from build123d import *

# Parameters (mm, degrees)
SKETCH_1_W          = 9.5
SKETCH_1_H          = 9.5
EXTRUDE_1_DEPTH     = 3
CUT_EXTRUDE_1_DEPTH = 1


with BuildPart() as part:
    # 草图1 → 凸台-拉伸1 (new body, symmetric)
    with BuildSketch(Plane.XY):
        with BuildLine():
            Line((-12, 0), (-12, 120))
            ThreePointArc((-12, 120), (0, 132), (12, 120))
            Line((12, 120), (12, 0))
            ThreePointArc((12, 0), (0, -12), (-12, 0))
        make_face()
        Rectangle(SKETCH_1_W, SKETCH_1_H, mode=Mode.SUBTRACT)
    extrude(amount=EXTRUDE_1_DEPTH, both=True)

    # 草图2 → 切除-拉伸1 (cut)
    with BuildSketch(Plane.XY.offset(3)):
        with BuildLine():
            Line((-6, 20), (-6, 120))
            ThreePointArc((-6, 120), (0, 126), (6, 120))
            Line((6, 120), (6, 20))
            ThreePointArc((6, 20), (0, 14), (-6, 20))
        make_face()
    cut_extrude_1 = extrude(amount=-CUT_EXTRUDE_1_DEPTH, mode=Mode.SUBTRACT)

    # 镜向1: 切除-拉伸1 across plane
    add(cut_extrude_1.mirror(Plane.XY), mode=Mode.SUBTRACT)


solid = part.part
The listing builds one solid part. Answer for the finished solid, in the listing's coordinates (mm). A direction names the side the tool comes from. Round coordinates to 2 decimals unless told otherwise and drop trailing zeros. Order: outer loops, then holes, each group sorted by start corner. A loop starts at its lowest first (then second) coordinate and runs counter-clockwise, first axis right, second up. Notation, with made-up numbers: (63, 88.5) - (73, 88.5) arc R12 ccw to (73, 98.5) - close; hole circle Ø1 at (73, -9.75). An arc over 180 degrees is marked (long way). Write item = value, one per line. Start each with the question number.
1) For a pull along X with two mould halves and no side action, classify faces 6 (the flat face through (-12, 59, 0)), 7 (the flat face through (0, 71, -2)), 8 (the flat face through (8, 61, -3)) as released by +X, released by -X, zero draft, split by the parting line, or undercut.
2) Given pin 1 (3.5 mm diameter, centred on x = -1, y = 55, fed in from +Z); pin 2 (5 mm diameter, centred on x = -5, y = 67, fed in from -Z); pin 3 (1 mm diameter, centred on x = -6, z = 2, fed in from -Y), each flat-ended and moving along its own axis, determine where each tip first touches the part or whether it passes through.
3) Section B-B, the plane x = 0 is taken. Write down the section's boundary in (y, z).
4) Section A-A, the plane z = 1.1 is taken. Write down the section's boundary in (x, y), plus the area to 3 significant figures.
5) Section D-D, the plane x = 8 is taken. Write down the section's boundary in (y, z).
6) Section C-C, the plane y = 44.5 is taken. Write down the section's boundary in (x, z).
7) For faces 1 (the cylindrical face through (0, -12, 0)), 2 (the cylindrical face through (0, 132, 0)), 3 (the flat face through (4.75, 0, 0)), 4 (the cylindrical face through (-0.1, 126, 2.5)), 5 (the cylindrical face through (0.1, 14, -2.5)), determine the directions among +Z, -Z, +X, -X, +Y, -Y from which every point of the face is accessible in a straight line to the end or side of a thin tool.
8) Straight lines are drawn through the part: L1, parallel to X at y = 35, z = -2.05; L2, parallel to Y at x = -4, z = -2.6; L3, parallel to Y at x = 0, z = 1.25. For each, find the intervals that lie inside material, in ascending order.
Results list:
q1.face_6 = released by -X
q1.face_7 = undercut
q1.face_8 = zero draft
q2.pin_1 = 2
q2.pin_2 = -3
q2.pin_3 = -10.67
q3.outline = (-12, -3) - (-4.75, -3) - (-4.75, 3) - (-12, 3) - close; (4.75, -3) - (14, -3) - (14, -2) - (126, -2) - (126, -3) - (132, -3) - (132, 3) - (126, 3) - (126, 2) - (14, 2) - (14, 3) - (4.75, 3) - close
q4.outline = (-12, 0) arc R12 ccw to (12, 0) - (12, 120) arc R12 ccw to (-12, 120) - close; hole (-4.75, -4.75) - (4.75, -4.75) - (4.75, 4.75) - (-4.75, 4.75) - close
q4.area = 3,240 mm^2
q5.outline = (-8.94, -3) - (128.94, -3) - (128.94, 3) - (-8.94, 3) - close
q6.outline = (-12, -3) - (-6, -3) - (-6, -2) - (6, -2) - (6, -3) - (12, -3) - (12, 3) - (6, 3) - (6, 2) - (-6, 2) - (-6, 3) - (-12, 3) - close
q7.face_1 = +Z, -Z, -Y
q7.face_2 = +Z, -Z, +Y
q7.face_3 = +Z, -Z
q7.face_4 = +Z
q7.face_5 = -Z
q8.L1 = -12 to -6, 6 to 12
q8.L2 = -11.31 to -4.75, 4.75 to 15.53, 124.47 to 131.31
q8.L3 = -12 to -4.75, 4.75 to 132
